Autodesk Inventor part; units mm, degrees
ref_plane "Work Plane1" through (0, 0, 100) normal (0, 0, 1) x (1, 0, 0)
ref_plane "Work Plane2" through (0, 0, 90) normal (0, 0, 1) x (1, 0, 0)
ref_plane "Work Plane3" through (10, 0, 0) normal (1, 0, 0) x (0, 1, 0)
sketch "Sketch1" plane through (0, 0, 0) normal (1, 0, 0) x (0, 1, 0)
  line L0 (0, 0) -> (0, 80)
  line L1 (0, 0) -> (25, 0)
  line L2 (25, 0) -> (25, 15)
  line L3 (25, 15) -> (2.5, 15) construction
  line L4 (2.5, 15) -> (2.5, 50) construction
  line L5 (2.5, 80) -> (0, 80)
  arc A0 (2.5, 50) -> (25, 15) centre (40.9722, 50) ccw
  line L6 (2.5, 50) -> (2.5, 80)
  dimension "d0" = 50
  dimension "d1" = 80
  dimension "d2" = 15
  dimension "d3" = 5
  dimension "d4" = 35
revolve "Revolution1" add sketch "Sketch1" angle 360 about axis through (0, 0, 0) along (0, 0, 1)
ref_plane "Work Plane1" through (0, 0, 100) normal (0, 0, 1) x (1, 0, 0)
sketch "Sketch3" plane through (0, 0, 100) normal (0, 0, 1) x (1, 0, 0)
  line L0 (-0.5, -0.5) -> (0.5, -0.5)
  line L1 (0.5, -0.5) -> (0.5, 0.5)
  line L2 (0.5, 0.5) -> (-0.5, 0.5)
  line L3 (-0.5, 0.5) -> (-0.5, -0.5)
  line L4 (-0.5, -0.5) -> (0.5, 0.5) construction
  line L5 (0.5, -0.5) -> (-0.5, 0.5) construction
  point P0 (0, 0)
  dimension "d7" = 1
  dimension "d8" = 1
ref_plane "Work Plane2" through (0, 0, 90) normal (0, 0, 1) x (1, 0, 0)
sketch "Sketch4" plane through (0, 0, 90) normal (0, 0, 1) x (1, 0, 0)
  line L0 (-2.5, -2.5) -> (2.5, -2.5)
  line L1 (2.5, -2.5) -> (2.5, 2.5)
  line L2 (2.5, 2.5) -> (-2.5, 2.5)
  line L3 (-2.5, 2.5) -> (-2.5, -2.5)
  line L4 (-2.5, -2.5) -> (2.5, 2.5) construction
  line L5 (2.5, -2.5) -> (-2.5, 2.5) construction
  point P0 (0, 0)
  dimension "d10" = 5
  dimension "d11" = 5
loft "Loft1" add profiles "Sketch4", "Sketch3" section 1 edges at (0, -2.5, 80)
sketch "Sketch5" plane through (0, 0, 0) normal (1, 0, 0) x (0, 1, 0)
  line L0 (1.7678, 80) -> (1.7678, 80)
  line L1 (1.7678, 80) -> (-1.7678, 80)
  line L2 (-1.7678, 80) -> (-1.7678, 80)
  line L3 (-1.7678, 80) -> (1.7678, 80)
  line L4 (-2.5, 50) -> (2.5, 50)
  line L5 (-1.5, 81.5) -> (1.5, 81.5)
  line L6 (1.5, 81.5) -> (1.5, 78.5)
  line L7 (1.5, 78.5) -> (-1.5, 78.5)
  line L8 (-1.5, 78.5) -> (-1.5, 81.5)
  line L9 (-1.7678, 80) -> (1.7678, 80)
  line L10 (-1.5, 81.5) -> (1.5, 78.5) construction
  line L11 (1.5, 81.5) -> (-1.5, 78.5) construction
  point P0 (0, 0)
  point P1 (0, 80)
  dimension "d18" = 3
  dimension "d19" = 3
ref_plane "Work Plane3" through (10, 0, 0) normal (1, 0, 0) x (0, 1, 0)
sketch "Sketch6" plane through (10, 0, 0) normal (1, 0, 0) x (0, 1, 0)
  line L0 (1.7678, 80) -> (1.7678, 80)
  line L1 (1.7678, 80) -> (-2.5, 80)
  line L2 (-2.5, 80) -> (-1.7678, 80)
  line L3 (-1.7678, 80) -> (1.7678, 80)
  line L4 (-2.5, 50) -> (2.5, 50)
  line L5 (-0.25, 80.25) -> (0.25, 80.25)
  line L6 (0.25, 80.25) -> (0.25, 79.75)
  line L7 (0.25, 79.75) -> (-0.25, 79.75)
  line L8 (-0.25, 79.75) -> (-0.25, 80.25)
  line L9 (-2.5, 80) -> (1.7678, 80)
  line L10 (-0.25, 80.25) -> (0.25, 79.75) construction
  line L11 (0.25, 80.25) -> (-0.25, 79.75) construction
  point P0 (0, 0)
  point P1 (0, 80)
  dimension "d21" = 0.5
  dimension "d22" = 0.5
loft "Loft2" add profiles "Sketch5", "Sketch6"
properties part number "EndEffector"
Read the model definition and answer for the solid it produces. Units are mm, in the model's axes. Give positions to 0.01 mm unless a question says otherwise; leave off trailing zeros. Loops run counter-clockwise (first coordinate to the right, second up) from the corner with the lowest first, then second, coordinate; pieces in that order, holes last. Notation, with made-up numbers: M 39,21.5 L 80,21.5 A20 cw 80,47.5 Z; hole C 58.25,54 d2. An arc over 180 degrees is marked long. Write each question's results on one line, items separated by ' | '.
1. Section B-B on z = 37 is taken. Give the vertices of the cut face in (x, y).
Values:
outline: C 0,0 d9.53
2. Section A-A on z = 57 is taken. Give the vertices of the cut face in (x, y), plus the area to 3 significant figures.
Values:
outline: C 0,0 d5 | area: 19.6 mm^2
3. The mould has two halves that part along Z. Classify faces 1 (the face through (0, 0, 0)), 2 (the face through (2.44, -0.54, 65.21)), 3 (the face through (-7.509, 23.846, 7.605)): pulls with the +Z half, pulls with the -Z half, needs draft (parallel to the pull), parting line crosses it, or undercut.
Values:
face 1: pulls with the -Z half | face 2: undercut | face 3: needs draft
4. Straight lines are drawn through the part: line 1 (Z direction, x = -2, y = 5.5); line 2 (Z direction, x = 11, y = 9); line 3 (X direction, y = 1.5, z = 88). For each, find the intervals that lie inside material, in ascending order. Write a range as [from, to].
Values:
line 1: z = [0, 34.29] | line 2: z = [0, 22.36] | line 3: x = [-2.62, 2.62]
5. Given pin 1 (2 mm diameter, centred on y = 0.5, z = 17.5, fed in from -X); pin 2 (6 mm diameter, centred on x = 10, y = 7.5, fed in from +Z); pin 3 (5 mm diameter, centred on x = -14, y = 16, fed in from +Z); pin 4 (1 mm diameter, centred on x = -11, y = -14.5, fed in from -Z), each flat-ended and moving along its own axis, determine where each tip first touches the part or whether it passes through.
Values:
pin 1: stops at x = -22.05 | pin 2: stops at z = 27.87 | pin 3: stops at z = 18.59 | pin 4: stops at z = 0
